```python
from build123d import *

# Parameters (mm, degrees)
SKETCH3_W           = 24
SKETCH3_H           = 24
BOSS_EXTRUDE1_DEPTH = 2
SKETCH4_W           = 3.021973807
SKETCH4_H           = 8
BOSS_EXTRUDE2_DEPTH = 15
SKETCH6_R           = 2.35
CUT_EXTRUDE1_DEPTH  = 3.2
SKETCH7_R           = 4
BOSS_EXTRUDE3_DEPTH = 2
SKETCH8_R           = 1
CUT_EXTRUDE2_DEPTH  = 2
SKETCH9_R           = 1.25
CUT_EXTRUDE3_DEPTH  = 0.3


with BuildPart() as part:
    # Sketch3 → Boss-Extrude1 (new body)
    with BuildSketch(Plane(origin=(0, 0, 0), x_dir=(1, 0, 0), z_dir=(0, 1, 0))):
        with Locations((-15.971223022, 1.424460432)):
            Rectangle(SKETCH3_W, SKETCH3_H)
    extrude(amount=BOSS_EXTRUDE1_DEPTH)

    # Sketch4 → Boss-Extrude2 (add)
    with BuildSketch(Plane(origin=(0, 2, 0), x_dir=(1, 0, 0), z_dir=(0, 1, 0))):
        with Locations((-26.460236118, -5.075539568)):
            Rectangle(SKETCH4_W, SKETCH4_H)
    extrude(amount=BOSS_EXTRUDE2_DEPTH)

    # Sketch6 → Cut-Extrude1 (cut)
    with BuildSketch(Plane(origin=(-24.949249215, 0, 0), x_dir=(0, 0, -1), z_dir=(1, 0, 0))):
        with Locations((-5.075539568, 13)):
            Circle(SKETCH6_R)
    extrude(amount=-CUT_EXTRUDE1_DEPTH, mode=Mode.SUBTRACT)

    # Sketch7 → Boss-Extrude3 (add)
    with BuildSketch(Plane.ZY.offset(27.971223022)):
        with Locations((5.075539568, 13)):
            Circle(SKETCH7_R)
    extrude(amount=BOSS_EXTRUDE3_DEPTH)

    # Sketch8 → Cut-Extrude2 (cut)
    with BuildSketch(Plane.ZY.offset(29.971223022)):
        with Locations((5.075539568, 13)):
            Circle(SKETCH8_R)
    extrude(amount=-CUT_EXTRUDE2_DEPTH, mode=Mode.SUBTRACT)

    # Sketch9 → Cut-Extrude3 (cut)
    with BuildSketch(Plane.ZY.offset(29.971223022)):
        with Locations((5.075539568, 13)):
            Circle(SKETCH9_R)
    extrude(amount=-CUT_EXTRUDE3_DEPTH, mode=Mode.SUBTRACT)


solid = part.part
```
The listing builds one solid part. Answer for the finished solid, in the listing's coordinates (mm). A direction names the side the tool comes from. Coordinates: 2 decimals unless noted, no trailing zeros. Order: outer loops, then holes, each group sorted by start corner. A loop starts at its lowest first (then second) coordinate and runs counter-clockwise, first axis right, second up. Notation, with made-up numbers: M 67.25,-34 L 99.25,-34 A8 cw 99.25,-25 Z; hole C -28,-37 d8. An arc over 180 degrees is marked long. Answer as a JSON object with one key per item and string values. Group by question number.
1. Section D-D on z = -3.75 is taken. Write down the section's boundary in (x, y).
2. A tool of negligible diameter and unlimited length cuts with its end or side. For faces 1 (the flat face through (-24.949, 9, 5)), 2 (the flat face through (-27.971, 16, 8)), 3 (the flat face through (-26, 9, 1.076)), 4 (the cylindrical face through (-28.96, 16.37, 7.23)), 5 (the cylindrical face through (-26.439, 10.706, 5.585)), from which of +Z, -Z, +X, -X, +Y, -Y can it reach the whole face along a straight path? Write none if from no direction.
3. Section A-A on x = -25.5 is taken. Write down the section's boundary in (y, z), then the cut area to 3 significant figures.
4. Straight lines are drawn through the part: line 1 (Y direction, x = -7.5, z = -5.75); line 2 (X direction, y = 6.5, z = 3.25); line 3 (X direction, y = 10, z = 3.75). For each, find the intervals that lie inside material, in ascending order.
5. Flat-ended cylindrical pins translate along their axes: P1, Ø6, axis at x = -19, y = 10.5, coming from the +Z side; P2, Ø4, axis at y = 13.5, z = 3, coming from the +X side; P3, Ø2.5, axis at y = 13, z = 4.5, coming from the +X side; P4, Ø4, axis at y = 4, z = 3.5, coming from the -X side. Find the tip coordinate at first contact, or state that the pin passes through.
6. Section C-C on y = 7.25 is taken. Write down the section's boundary in (x, z), then the cut area to 3 significant figures.
7. Section B-B on z = 3.5 is taken. Write down the section's boundary in (x, y), then the cut area to 3 significant figures.
Values follow:
{
 "1": {"outline": "M -27.97,0 L -3.97,0 L -3.97,2 L -27.97,2 Z"},
 "2": {"face 1": "+Z, -Z, +X, +Y", "face 2": "+Z, -X, +Y", "face 3": "-Z, +X, -X, +Y", "face 4": "-X", "face 5": "+X"},
 "3": {"outline": "M 0,-13.42 L 2,-13.42 L 2,1.08 L 17,1.08 L 17,9.08 L 2,9.08 L 2,10.58 L 0,10.58 Z; hole C 13,5.08 d4.7", "area": "151 mm2"},
 "4": {"line 1": "0 to 2", "line 2": "-27.97 to -24.95", "line 3": "-29.97 to -24.95"},
 "5": {"P1": "through", "P2": "x = -24.95", "P3": "x = -27.97", "P4": "x = -27.97"},
 "6": {"outline": "M -27.97,1.08 L -24.95,1.08 L -24.95,9.08 L -27.97,9.08 Z", "area": "24.2 mm2"},
 "7": {"outline": "M -29.97,9.32 L -27.97,9.32 L -27.97,0 L -3.97,0 L -3.97,2 L -24.95,2 L -24.95,11.26 L -27.97,11.26 L -27.97,14.74 L -24.95,14.74 L -24.95,17 L -27.97,17 L -27.97,16.68 L -29.97,16.68 Z", "area": "97.5 mm2"}
}
